Autodesk Inventor part; units mm, degrees
ref_plane "YZ Plane" through (0, 0, 0) normal (1, 0, 0) x (0, 1, 0)
ref_plane "XZ Plane" through (0, 0, 0) normal (0, 1, 0) x (-1, 0, 0)
ref_plane "XY Plane" through (0, 0, 0) normal (0, 0, 1) x (1, 0, 0)
sketch "Sketch1" plane through (0, 0, 0) normal (0, 0, 1) x (1, 0, 0)
  line L0 (0, 0) -> (0, 66)
  line L1 (0, 66) -> (36, 66)
  line L2 (36, 66) -> (36, 0)
  line L3 (36, 0) -> (0, 0)
  dimension "d0" = 66
  dimension "d1" = 36
extrude "Extrusion1" add sketch "Sketch1" along normal blind 3
sketch "Sketch2" plane through (0, 0, 3) normal (0, 0, 1) x (1, 0, 0)
  line L0 (36, 66) -> (0, 66)
  line L1 (36, 66) -> (43, 66)
  line L2 (43, 66) -> (43, 0)
  line L3 (36, 0) -> (36, 66)
  line L4 (43, 0) -> (36, 0)
  line L5 (39.5, 66) -> (39.5, 59.5)
  line L6 (39.5, 0) -> (39.5, 6.5)
  line L7 (43, 33) -> (39.5, 33)
  circle A0 centre (39.5, 33) radius 1.5
  circle A1 centre (39.5, 59.5) radius 1.5
  circle A2 centre (39.5, 6.5) radius 1.5
  line L8 (18, 66) -> (18, 77.4734)
  line L9 (0, 66) -> (-7, 66)
  line L10 (-7, 66) -> (-7, 0)
  line L11 (-7, 0) -> (0, 0)
  line L12 (-3.5, 66) -> (-3.5, 59.5)
  line L13 (-3.5, 0) -> (-3.5, 6.5)
  line L14 (-7, 33) -> (-3.5, 33)
  circle A3 centre (-3.5, 33) radius 1.5
  circle A4 centre (-3.5, 59.5) radius 1.5
  circle A5 centre (-3.5, 6.5) radius 1.5
  line L15 (36, 0) -> (36, 66)
  line L16 (36, 66) -> (0, 66)
  line L17 (0, 66) -> (0, 0)
  line L18 (0, 0) -> (36, 0)
  dimension "d4" = 7
  dimension "d5" = 6.5
  dimension "d6" = 6.5
  dimension "d7" = 3
  dimension "d8" = 3
  dimension "d9" = 3
extrude "Extrusion2" add sketch "Sketch2" against normal blind 3 contours L1 L2 L4 L3 | L17 L11 L10 L9
properties part number "middle steel plate"
Input: part model. Units: mm. Frame: model coordinates. Give positions to 0.01 mm unless a question says otherwise; leave off trailing zeros. Order: outer loops, then holes, each group sorted by start corner. A loop starts at its lowest first (then second) coordinate and runs counter-clockwise, first axis right, second up.
1. Pin query (flat end, axial travel): pin 1 (2.5 mm diameter, centred on x = 39.5, y = 33, fed in from -Z). Return the tip coordinate at first contact, or that it passes through.
Derived:
pin 1: passes through
2. Mould query, pull axis Y, two halves, no side actions, for faces 1 (the cylindrical face through (-3.695, 60.987, 1.521)), 2 (the flat face through (-7, 33, 2)), 3 (the flat face through (18, 0, 1)), 4 (the cylindrical face through (-2.81, 31.67, 1.52)). Classes: released by +Y, released by -Y, zero draft, split by the parting line, or undercut.
Derived:
face 1: undercut
face 2: zero draft
face 3: released by -Y
face 4: undercut
3. Section B-B on y = 59.5. Return the cut outline in (x, z).
Derived:
outline: (-7, 0) - (-5, 0) - (-5, 3) - (-7, 3) - close; (-2, 0) - (38, 0) - (38, 3) - (-2, 3) - close; (41, 0) - (43, 0) - (43, 3) - (41, 3) - close
4. Section A-A on x = -3.5. Return the cut outline in (y, z), and give its area (3 significant figures).
Derived:
outline: (0, 0) - (5, 0) - (5, 3) - (0, 3) - close; (8, 0) - (31.5, 0) - (31.5, 3) - (8, 3) - close; (34.5, 0) - (58, 0) - (58, 3) - (34.5, 3) - close; (61, 0) - (66, 0) - (66, 3) - (61, 3) - close
area: 171 mm2
5. Material intervals for L1, parallel to Y at x = -3.5, z = 2, sorted ascending.
Derived:
L1: y = 0 to 5, 8 to 31.5, 34.5 to 58, 61 to 66
